Print and shaded views of the part. All mm, measured from the part's lowest x, y and z. Give positions to 0.01 mm unless a question says otherwise; leave off trailing zeros. Order: outer loops, then holes, each group sorted by start corner. A loop starts at its lowest first (then second) coordinate and runs counter-clockwise, first axis right, second up. Notation, with made-up numbers: (41, 6.5) - (46, 6.5) arc R14 ccw to (46, 28.5) - close; hole circle Ø5 at (7.5, 57.25). An arc over 180 degrees is marked (long way). Answer in a Markdown table with one row per item.
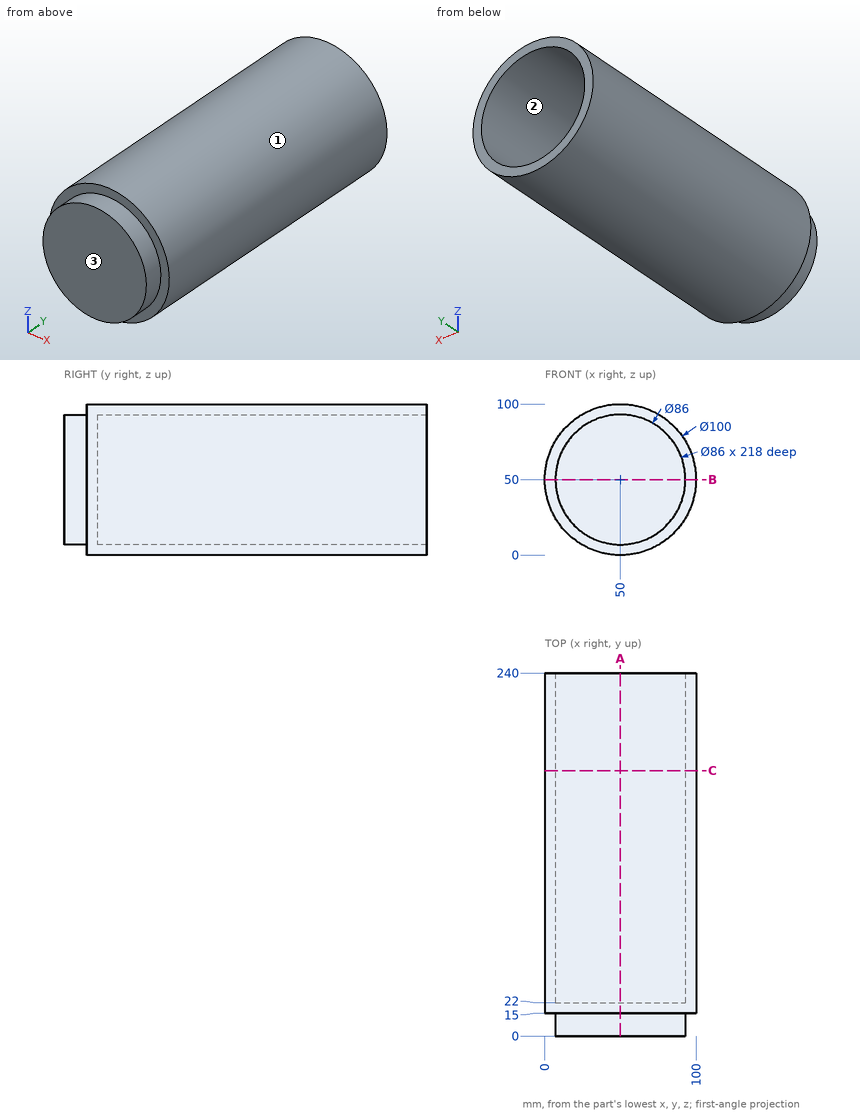
1. Cut at C-C on y = 175.5. Write the cut outline in (x, z).
Check result:
| item | result |
|---|---|
| outline | circle Ø100 at (50, 50); hole circle Ø86 at (50, 50) |
2. Probe line 1 (X direction, y = 181, z = 50); line 2 (Y direction, x = 43.5, z = 81); line 3 (Z direction, x = 31, y = 202). List the from-to ranges inside material, lowest first.
Check result:
| item | result |
|---|---|
| line 1 | x = 0 to 7, 93 to 100 |
| line 2 | y = 0 to 22 |
| line 3 | z = 3.75 to 11.43, 88.57 to 96.25 |
3. Two-plate mould, pull along Z, no slides. Class the marked faces 1, 2 and 3: +Z half, -Z half, draft (parallel to the pull), parting line (faces both ways), or undercut.
Check result:
| item | result |
|---|---|
| face 1 | parting line |
| face 2 | undercut |
| face 3 | draft |
4. Cut at B-B on z = 50. Write the cut outline in (x, y).
Check result:
| item | result |
|---|---|
| outline | (0, 15) - (7, 15) - (7, 0) - (93, 0) - (93, 15) - (100, 15) - (100, 240) - (93, 240) - (93, 22) - (7, 22) - (7, 240) - (0, 240) - close |
5. Drop flat-ended pins along their axis: P1, Ø5, axis at x = 87, y = 49, coming from the +Z side; P2, Ø3, axis at y = 201.5, z = 18.5, coming from the +X side; P3, Ø4, axis at y = 193.5, z = 41.5, coming from the +X side. Give the stop position or say it passes through.
Check result:
| item | result |
|---|---|
| P1 | stops at z = 86.19 |
| P2 | stops at x = 90 |
| P3 | stops at x = 99.58 |
6. Cut at A-A on x = 50. Write the cut outline in (y, z), and give its area (3 significant figures).
Check result:
| item | result |
|---|---|
| outline | (0, 7) - (15, 7) - (15, 0) - (240, 0) - (240, 7) - (22, 7) - (22, 93) - (240, 93) - (240, 100) - (15, 100) - (15, 93) - (0, 93) - close |
| area | 5,040 mm² |
